Design review of the part built by this model. Coordinates are the model's own, in mm. A direction names the side the tool comes from. Round coordinates to 2 decimals unless told otherwise and drop trailing zeros. Loops run counter-clockwise (first coordinate to the right, second up) from the corner with the lowest first, then second, coordinate; pieces in that order, holes last. Notation, with made-up numbers: (32, 62.25) - (75, 62.25) arc R19 ccw to (75, 85.25) - close; hole circle Ø1 at (55, -19). An arc over 180 degrees is marked (long way). Answer as CSV lines item,"result". Start each with the question number.
(1) Consider section B-B (x = 10). Give the boundary of the cut face in (y, z).
(2) Mouldability with a two-part tool opening along X and no side actions: class faces 5 (the flat face through (-15, 3, 75)), 6 (the flat face through (12.5, 3, 78)), 7 (the cylindrical face through (10.55, 3.13, -66.28)), 8 (the cylindrical face through (-9.45, 3.13, -66.28)) as released by +X, released by -X, zero draft, split by the parting line, or undercut.
(3) For P1, Ø3, axis at y = 3.5, z = -77.5, coming from the -X side; P2, Ø3, axis at y = 4.5, z = -77.5, coming from the +X side; P3, Ø3.5, axis at x = -10, z = 64.54, coming from the -Y side; P4, Ø2.5, axis at x = -14, y = 3, coming from the -Z side, all flat-tipped, find the tip position at first contact; note any pin that passes through.
(4) For faces 1 (the flat face through (-12.5, 3, 78)), 2 (the flat face through (15, 3, -75)), 3 (the flat face through (15, 3, 75)), 4 (the flat face through (-12.5, 3, -78)), list the 3-axis set-ups (+Z, -Z, +X, -X, +Y, -Y) from which the entire face can be reached by the end or side of a thin tool; tool diameter is ignored.
(5) Consider section C-C (y = 1.25). Give the boundary of the cut face in (x, z).
(6) Consider section A-A (z = 10). Give the boundary of the cut face in (x, y), and give its area (3 significant figures).
(7) Wall thickness on L1, parallel to X at y = 5.25, z = -10; L2, parallel to Z at x = 10.5, y = 3.5; L3, parallel to Z at x = -5, y = 2.25: over which ranges is each line inside the solid? List them lowest first.
(8) Consider section D-D (x = -6.5). Give the boundary of the cut face in (y, z).
from build123d import *

# Parameters (mm, degrees)
SKETCH1_W             = 35
SKETCH1_H             = 150
BOSS_EXTRUDE1_DEPTH   = 6.35
SKETCH2_W             = 25
SKETCH2_H             = 6.35
BOSS_EXTRUDE2_DEPTH   = 6.35
F_6_CLEARANCE_HOLE1_D = 3.6576
M5_CLEARANCE_HOLE1_D  = 5.3


with BuildPart() as part:
    # Sketch1 → Boss-Extrude1 (new body)
    with BuildSketch(Plane(origin=(0, 0, 0), x_dir=(1, 0, 0), z_dir=(0, 1, 0))):
        Rectangle(SKETCH1_W, SKETCH1_H)
    extrude(amount=BOSS_EXTRUDE1_DEPTH)

    # Sketch2 → Boss-Extrude2 (add)
    with BuildSketch(Plane(origin=(0, 6.35, 0), x_dir=(1, 0, 0), z_dir=(0, 1, 0))):
        with Locations((0, -78.175)):
            Rectangle(SKETCH2_W, SKETCH2_H)
        with Locations((0, 78.175)):
            Rectangle(SKETCH2_W, SKETCH2_H)
    extrude(amount=-BOSS_EXTRUDE2_DEPTH)

    # #6 Clearance Hole1 (through all)
    with Locations(Plane(origin=(-10, 6.35, -64.5352), x_dir=(0, 0, 1), z_dir=(0, 1, 0))):
        with Locations((0, 0), (0, 20), (129.0704, 20), (129.0704, 0)):
            Hole(F_6_CLEARANCE_HOLE1_D / 2)

    # M5 Clearance Hole1 (through all)
    with Locations(Plane(origin=(-6.5, 6.35, 10), x_dir=(0, 0, 1), z_dir=(0, 1, 0))):
        with Locations((0, 0), (-20, 0)):
            Hole(M5_CLEARANCE_HOLE1_D / 2)


solid = part.part
Determined:
1,outline,"(0, -81.35) - (6.35, -81.35) - (6.35, -66.36) - (0, -66.36) - close; (0, -62.71) - (6.35, -62.71) - (6.35, 62.71) - (0, 62.71) - close; (0, 66.36) - (6.35, 66.36) - (6.35, 81.35) - (0, 81.35) - close"
2,face 5,"zero draft"
2,face 6,"released by +X"
2,face 7,"undercut"
2,face 8,"undercut"
3,P1,"stops at x = -12.5"
3,P2,"stops at x = 12.5"
3,P3,"passes through"
3,P4,"stops at z = -75"
4,face 1,"+Z, -X, +Y, -Y"
4,face 2,"-Z, +X, +Y, -Y"
4,face 3,"+Z, +X, +Y, -Y"
4,face 4,"-Z, -X, +Y, -Y"
5,outline,"(-17.5, -75) - (-12.5, -75) - (-12.5, -81.35) - (12.5, -81.35) - (12.5, -75) - (17.5, -75) - (17.5, 75) - (12.5, 75) - (12.5, 81.35) - (-12.5, 81.35) - (-12.5, 75) - (-17.5, 75) - close; hole circle Ø3.66 at (-10, -64.54); hole circle Ø3.66 at (-10, 64.54); hole circle Ø5.3 at (-6.5, -10); hole circle Ø5.3 at (-6.5, 10); hole circle Ø3.66 at (10, -64.54); hole circle Ø3.66 at (10, 64.54)"
6,outline,"(-17.5, 0) - (-9.15, 0) - (-9.15, 6.35) - (-17.5, 6.35) - close; (-3.85, 0) - (17.5, 0) - (17.5, 6.35) - (-3.85, 6.35) - close"
6,area,"189 mm^2"
7,L1,"x = -17.5 to -9.15, -3.85 to 17.5"
7,L2,"z = -81.35 to -66.29, -62.78 to 62.78, 66.29 to 81.35"
7,L3,"z = -81.35 to -12.18, -7.82 to 7.82, 12.18 to 81.35"
8,outline,"(0, -81.35) - (6.35, -81.35) - (6.35, -12.65) - (0, -12.65) - close; (0, -7.35) - (6.35, -7.35) - (6.35, 7.35) - (0, 7.35) - close; (0, 12.65) - (6.35, 12.65) - (6.35, 81.35) - (0, 81.35) - close"
